Could you check a few things on this model? Use its own coordinates, in mm. A direction names the side the tool comes from. Give positions to 0.01 mm unless a question says otherwise; leave off trailing zeros. Write each loop counter-clockwise with the first axis right and the second up, starting at its lowest first coordinate (ties: lowest second). Pieces come first, ordered by that corner, then holes. Notation, with made-up numbers: (8.5, 59) -> (37.5, 59) arc R15 ccw to (37.5, 68) -> close; hole circle Ø2 at (12.25, -8). An arc over 180 degrees is marked (long way). Write item = value, one per line. Start each with the question number.
```python
from build123d import *

# Parameters (mm, degrees)
SKETCH1_R           = 3.96875
BOSS_EXTRUDE1_DEPTH = 22.225
CHAMFER1_SIZE       = 0.508
CUT_EXTRUDE1_START  = 0.7366
SKETCH2_R           = 3.96875
SKETCH2_R_2         = 3.175
CUT_EXTRUDE1_DEPTH  = 0.7366


with BuildPart() as part:
    # Sketch1 → Boss-Extrude1 (new, symmetric)
    with BuildSketch(Plane(origin=(0, 0, 0), x_dir=(0, 0, -1), z_dir=(1, 0, 0))):
        Circle(SKETCH1_R)
    extrude(amount=BOSS_EXTRUDE1_DEPTH, both=True)

    # Chamfer1
    chamfer1_edges = [part.edges().sort_by_distance(p)[0] for p in [
        (-22.225, 0, 3.96875),
        (22.225, 0, 3.96875),
    ]]
    chamfer(chamfer1_edges, length=CHAMFER1_SIZE)

    # Sketch2 → Cut-Extrude1 (cut)
    with BuildSketch(Plane(origin=(20.6375, 0, 0), x_dir=(0, 0, -1), z_dir=(1, 0, 0)).offset(CUT_EXTRUDE1_START)):
        Circle(SKETCH2_R)
        Circle(SKETCH2_R_2, mode=Mode.SUBTRACT)
    cut_extrude1 = extrude(amount=-CUT_EXTRUDE1_DEPTH, mode=Mode.SUBTRACT)

    # Mirror1: Cut-Extrude1 across plane
    add(cut_extrude1.mirror(Plane(origin=(0, 0, 0), x_dir=(0, 0, 1), z_dir=(1, 0, 0))), mode=Mode.SUBTRACT)


solid = part.part
```
(1) On a 3-axis mill with a long thin cutter (end or side, diameter ignored), from which of +Z, -Z, +X, -X, +Y, -Y can I reach the whole of each face in a straight line? I mean faces 1 (the flat face through (-22.225, 0, 0)), 2 (the flat face through (-20.638, 3, 2)). Say none if no direction works.
(2) Imagine slicing it at A-A (x = -7.5). Please give me the cut outline in (y, z), then the cut area to 3 significant figures.
(3) If I drill on line 1 along X through (y, z) = (2.75, 2.75); line 2 along Y through (x, z) = (-20, -0.25); line 3 along Z through (x, y) = (5.5, -1), over which ranges is the centre line in solid material (lowest first)? Write a range as from..to.
(4) We'd pull the mould along X, two halves only. Please class faces 3 (the flat face through (22.225, 0, 0)), 4 (the cylindrical face through (0.289, -3.874, 0.86)), 5 (the flat face through (-21.374, 3, 2)): released by +X, released by -X, zero draft, split by the parting line, or undercut.
(5) I'm going to push flat-ended pins straight in: pin 1 (1.5 mm diameter, centred on x = 4.5, y = 2.5, fed in from +Z); pin 2 (2 mm diameter, centred on x = 13.5, z = 2.5, fed in from +Y); pin 3 (1.5 mm diameter, centred on x = 15.5, z = -2, fed in from -Y). Where does each tip first touch, or does it pass through?
Answers below:
q1.face_1 = +Z, -Z, -X, +Y, -Y
q1.face_2 = none
q2.outline = circle Ø7.94 at (0, 0)
q2.area = 49.5 mm^2
q3.line_1 = -21.8..-21.37, -20.64..20.64, 21.37..21.8
q3.line_2 = -3.96..3.96
q3.line_3 = -3.84..3.84
q4.face_3 = released by +X
q4.face_4 = zero draft
q4.face_5 = undercut
q5.pin_1 = 3.56
q5.pin_2 = 3.67
q5.pin_3 = -3.77
